Geometry: see drawing. Coordinates: mm, zero at the bounding-box minimum. A direction names the side the tool comes from. Coordinates: 2 decimals unless noted, no trailing zeros. Loops run counter-clockwise (first coordinate to the right, second up) from the corner with the lowest first, then second, coordinate; pieces in that order, holes last. Notation, with made-up numbers: (19, 25) -> (49, 25) arc R31 cw to (49, 62) -> close; hole circle Ø1 at (-9.75, 71.5). An arc over 180 degrees is marked (long way). Answer as a JSON object with one key per item and string values.
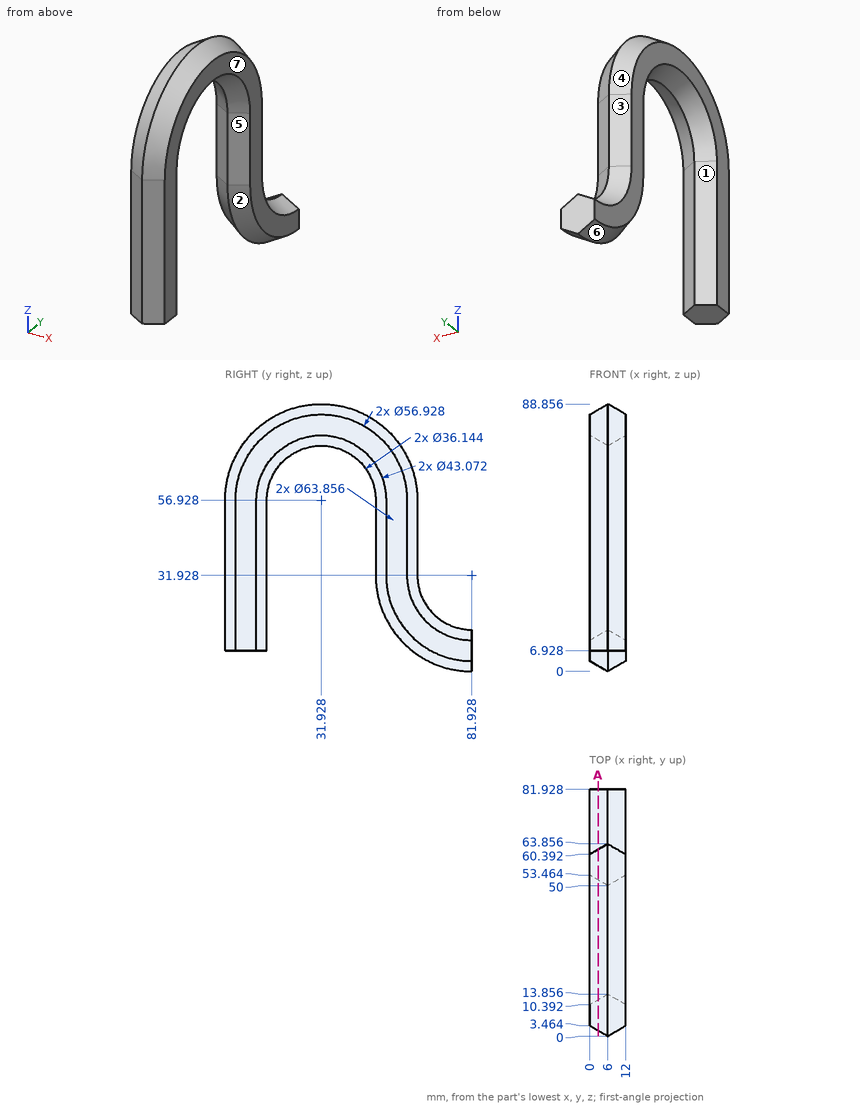
1. Access query for the marked faces 1, 2 and 3. Directions: +Z, -Z, +X, -X, +Y, -Y. A direction counts if a zero-diameter tool reaches every point of the face in a straight line with its end or side. Return the directions, or none.
Reply:
{"face 1": "-Z, -X", "face 2": "-Z, +X", "face 3": "+Z, -X, +Y"}
2. Mould query, pull axis Y, two halves, no side actions, for the marked faces 4, 5, 6 and 7. Classes: pulls with the +Y half, pulls with the -Y half, needs draft (parallel to the pull), parting line crosses it, or undercut.
Reply:
{"face 4": "parting line crosses it", "face 5": "undercut", "face 6": "undercut", "face 7": "needs draft"}
3. Line query: line 1 along Y through (x, z) = (1, 44) (1 decimal); line 2 along Y through (x, z) = (8.25, 43.5); line 3 along X through (y, z) = (62, 34) (1 decimal). Output: solid intervals per line, ascending.
Reply:
{"line 1": "y = 2.9 to 11, 52.9 to 61", "line 2": "y = 1.3 to 12.56, 51.3 to 62.56", "line 3": "x = 2.8 to 9.2"}
4. Pin query (flat end, axial travel): P1, Ø1, axis at x = 5, z = 44, coming from the +Y side; P2, Ø5, axis at x = 1.5, z = 55, coming from the -Y side (1 decimal); P3, Ø1, axis at x = 9, y = 59.5, coming from the +Z side (1 decimal). Return the tip coordinate at first contact, or that it passes through.
Reply:
{"P1": "stops at y = 63.57", "P2": "stops at y = 1.2", "P3": "stops at z = 70.5"}
5. Section query A-A (x = 2.75). Return loops of the section in (y, z).
Reply:
{"outline": "(1.88, 6.93) -> (11.98, 6.93) -> (11.98, 56.93) arc R19.95 cw to (51.88, 56.93) -> (51.88, 31.93) arc R30.05 ccw to (81.93, 1.88) -> (81.93, 11.98) arc R19.95 cw to (61.98, 31.93) -> (61.98, 56.93) arc R30.05 ccw to (1.88, 56.93) -> close"}
